```python
from build123d import *

# Parameters (mm, degrees)
SKETCH_1_W          = 5
SKETCH_1_H          = 126
EXTRUDE_1_DEPTH     = 5
SKETCH_2_R          = 1
CUT_EXTRUDE_1_DEPTH = 5
SKETCH_3_R          = 1
CUT_EXTRUDE_2_DEPTH = 5


with BuildPart() as part:
    # 草图1 → 凸台-拉伸1 (new body)
    with BuildSketch(Plane.XY):
        with Locations((-2.5, 63)):
            Rectangle(SKETCH_1_W, SKETCH_1_H)
    extrude(amount=EXTRUDE_1_DEPTH)

    # 草图2 → 切除-拉伸1 (cut)
    with BuildSketch(Plane.XY.offset(5)):
        with Locations((-2.5, 116)):
            Circle(SKETCH_2_R)
        with Locations((-2.5, 10)):
            Circle(SKETCH_2_R)
    extrude(amount=-CUT_EXTRUDE_1_DEPTH, mode=Mode.SUBTRACT)

    # 草图3 → 切除-拉伸2 (cut)
    with BuildSketch(Plane(origin=(0, 0, 0), x_dir=(0, 0, -1), z_dir=(1, 0, 0))):
        with Locations((-2.5, 106)):
            Circle(SKETCH_3_R)
        with Locations((-2.5, 20)):
            Circle(SKETCH_3_R)
    extrude(amount=-CUT_EXTRUDE_2_DEPTH, mode=Mode.SUBTRACT)


solid = part.part
```
Work out the finished part from the listing and answer in its coordinate system (mm). Coordinates: 2 decimals unless noted, no trailing zeros. Loops run counter-clockwise (first coordinate to the right, second up) from the corner with the lowest first, then second, coordinate; pieces in that order, holes last. Notation, with made-up numbers: (-23.75, 76) - (-6.75, 76) arc R13 ccw to (-6.75, 81) - close; hole circle Ø8 at (14.5, 5.25). An arc over 180 degrees is marked (long way). Use a Markdown table: item, result.
Item 1: Consider probe 1 along Y at (x, z) = (-2.5, 3.85); probe 2 along X at (y, z) = (116, 3.1); probe 3 along Z at (x, y) = (-3.05, 106). Determine where each line is inside the solid, lowest interval first. Write a range as from..to.
Evaluation:
| item | result |
|---|---|
| probe 1 | y = 0..9, 11..115, 117..126 |
| probe 2 | x = -5..-3.5, -1.5..0 |
| probe 3 | z = 0..1.5, 3.5..5 |
Item 2: Find section B-B, the plane x = -2.5. Determine the outline of the cut face in (y, z).
Evaluation:
| item | result |
|---|---|
| outline | (0, 0) - (9, 0) - (9, 5) - (0, 5) - close; (11, 0) - (115, 0) - (115, 5) - (11, 5) - close; (117, 0) - (126, 0) - (126, 5) - (117, 5) - close; hole circle Ø2 at (20, 2.5); hole circle Ø2 at (106, 2.5) |
Item 3: Find section A-A, the plane z = 2.5. Determine the outline of the cut face in (x, y).
Evaluation:
| item | result |
|---|---|
| outline | (-5, 0) - (0, 0) - (0, 19) - (-5, 19) - close; (-5, 21) - (0, 21) - (0, 105) - (-5, 105) - close; (-5, 107) - (0, 107) - (0, 126) - (-5, 126) - close; hole circle Ø2 at (-2.5, 10); hole circle Ø2 at (-2.5, 116) |
Item 4: The mould has two halves that part along X. Classify faces 1 (the flat face through (-3, 126, 2)), 2 (the flat face through (-5, 62, 2)), 3 (the cylindrical face through (-2.63, 10.99, 2.54)): +X half, -X half, draft (parallel to the pull), parting line (faces both ways), or undercut.
Evaluation:
| item | result |
|---|---|
| face 1 | draft |
| face 2 | -X half |
| face 3 | undercut |
